Part model, mm, in its own coordinate system. A direction names the side the tool comes from. Give positions to 0.01 mm unless a question says otherwise; leave off trailing zeros. Order: outer loops, then holes, each group sorted by start corner. A loop starts at its lowest first (then second) coordinate and runs counter-clockwise, first axis right, second up. Notation, with made-up numbers: M -36.5,-24 L 1.5,-24 A22 ccw 1.5,7 Z; hole C -31,13.5 d2. An arc over 180 degrees is marked long. Return JSON: item names as keys, results as strings.
from build123d import *

# Parameters (mm, degrees)
SKIZZE5_R                       = 1.52
AUFSATZ_LINEAR_AUSTRAGEN3_DEPTH = 30
SCHNITT_LINEAR_AUSTRAGEN1_DEPTH = 10


with BuildPart() as part:
    # Skizze5 → Aufsatz-Linear austragen3 (new body)
    with BuildSketch(Plane(origin=(0, 0, 0), x_dir=(0, 0, -1), z_dir=(1, 0, 0))):
        with BuildLine():
            Line((-11.555611309, 6.111130946), (-11.555611309, 4.111130946))
            Line((-11.555611309, 4.111130946), (9.717875997, 4.111130946))
            Line((9.717875997, 4.111130946), (9.717875997, 1.111130946))
            ThreePointArc((9.717875997, 1.111130946), (10.010769216, 0.404024165), (10.717875997, 0.111130946))
            Line((10.717875997, 0.111130946), (13.717875997, 0.111130946))
            ThreePointArc((13.717875997, 0.111130946), (14.424982778, 0.404024165), (14.717875997, 1.111130946))
            Line((14.717875997, 1.111130946), (14.717875997, 6.111130946))
            Line((14.717875997, 6.111130946), (14.217875997, 6.111130946))
            Line((14.217875997, 6.111130946), (-11.555611309, 6.111130946))
        make_face()
        with Locations((12.217875997, 2.111130946)):
            Circle(SKIZZE5_R, mode=Mode.SUBTRACT)
    extrude(amount=AUFSATZ_LINEAR_AUSTRAGEN3_DEPTH)

    # Skizze6 → Schnitt-Linear austragen1 (cut)
    with BuildSketch(Plane(origin=(0, 6.111130946, 0), x_dir=(1, 0, 0), z_dir=(0, 1, 0))):
        with BuildLine():
            Line((3.364391914, -3.782124003), (3.364391914, 2.217875997))
            ThreePointArc((3.364391914, 2.217875997), (4.914391914, 3.767875997), (6.464391914, 2.217875997))
            Line((6.464391914, 2.217875997), (6.464391914, -3.782124003))
            ThreePointArc((6.464391914, -3.782124003), (4.914391914, -5.332124003), (3.364391914, -3.782124003))
        make_face()
        with BuildLine():
            Line((26.635608086, -3.782124003), (26.635608086, 2.217875997))
            ThreePointArc((26.635608086, 2.217875997), (25.085608086, 3.767875997), (23.535608086, 2.217875997))
            Line((23.535608086, 2.217875997), (23.535608086, -3.782124003))
            ThreePointArc((23.535608086, -3.782124003), (25.085608086, -5.332124003), (26.635608086, -3.782124003))
        make_face()
    extrude(amount=-SCHNITT_LINEAR_AUSTRAGEN1_DEPTH, mode=Mode.SUBTRACT)


solid = part.part
Q1. Band-saw the part on D-D (z = -12.5). Give the cut face in (x, y), then the cut area to 3 significant figures.
Established:
{"outline": "M 0,0.11 L 30,0.11 L 30,0.62 L 0,0.62 Z; M 0,3.6 L 30,3.6 L 30,6.11 L 0,6.11 Z", "area": "90.4 mm²"}
Q2. Two-plate mould, pull along Z, no slides. Class faces 1 (the flat face through (15, 4, -14.718)), 2 (the cylindrical face through (25.05, 5.13, 5.33)), 3 (the flat face through (15, 6.111, -2)): +Z half, -Z half, draft (parallel to the pull), parting line (faces both ways), or undercut.
Established:
{"face 1": "-Z half", "face 2": "undercut", "face 3": "draft"}
Q3. Pin check, flat tips, straight feed: pin 1 (1 mm diameter, centred on y = 5, z = 2, fed in from -X); pin 2 (10 mm diameter, centred on x = 23, z = 7.5, fed in from -Y); pin 3 (0.9 mm diameter, centred on x = 21.5, y = 3, fed in from +Z). Stop position of each tip, or through.
Established:
{"pin 1": "stops at x = 0", "pin 2": "stops at y = 4.11", "pin 3": "stops at z = -9.72"}
Q4. Band-saw the part on B-B (y = 4.6). Give the cut face in (x, z), then the cut area to 3 significant figures.
Established:
{"outline": "M 0,-14.72 L 30,-14.72 L 30,11.56 L 0,11.56 Z; hole M 3.36,-2.22 A1.55 ccw 6.46,-2.22 L 6.46,3.78 A1.55 ccw 3.36,3.78 Z; hole M 23.54,-2.22 A1.55 ccw 26.64,-2.22 L 26.64,3.78 A1.55 ccw 23.54,3.78 Z", "area": "736 mm²"}
Q5. Band-saw the part on A-A (z = 1.75). Give the cut face in (x, y), then the cut area to 3 significant figures.
Established:
{"outline": "M 0,4.11 L 3.36,4.11 L 3.36,6.11 L 0,6.11 Z; M 6.46,4.11 L 23.54,4.11 L 23.54,6.11 L 6.46,6.11 Z; M 26.64,4.11 L 30,4.11 L 30,6.11 L 26.64,6.11 Z", "area": "47.6 mm²"}
Q6. Band-saw the part on C-C (x = 27). Give the cut face in (y, z).
Established:
{"outline": "M 0.11,-13.72 A1 ccw 1.11,-14.72 L 6.11,-14.72 L 6.11,11.56 L 4.11,11.56 L 4.11,-9.72 L 1.11,-9.72 A1 ccw 0.11,-10.72 Z; hole C 2.11,-12.22 d3.04"}
Q7. 3-axis set-ups, long thin cutter, end or side, ignore diameter. For faces 4 (the flat face through (23.536, 5, 1)), 5 (the flat face through (15, 0.111, -12)), 6 (the flat face through (15, 4.111, 1)): which of +Z, -Z, +X, -X, +Y, -Y reach the whole face in a straight line?
Established:
{"face 4": "+Y, -Y", "face 5": "+Z, -Z, +X, -X, -Y", "face 6": "+Z, +X, -X, -Y"}
Q8. Probe line 1 along Z through (x, y) = (4.25, 4.75); line 2 along Y through (x, z) = (27.5, -4.5); line 3 along Z through (x, y) = (7.25, 3.3). List the from-to ranges inside material, lowest first.
Established:
{"line 1": "z = -14.72 to -3.62, 5.18 to 11.56", "line 2": "y = 4.11 to 6.11", "line 3": "z = -14.72 to -13.16, -11.27 to -9.72"}
